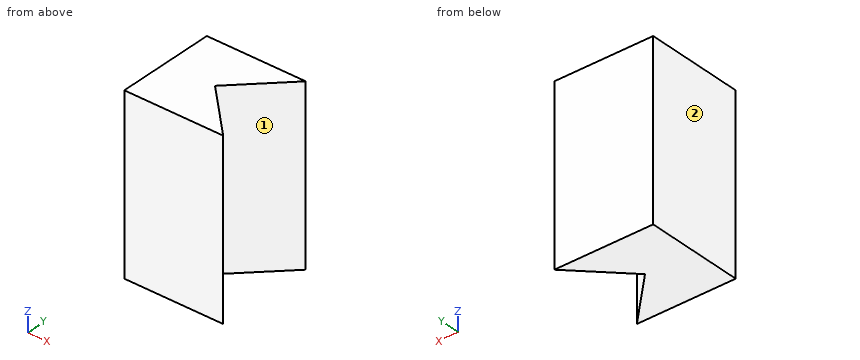
from build123d import *

# Parameters (mm, degrees)
F0_W     = 101.6
F0_H     = 101.6
F1_DEPTH = 177.8
F3_DEPTH = 177.8


with BuildPart() as f1:
    # F0 (on Top) → F1 (new body)
    with BuildSketch(Plane.XY):
        Rectangle(F0_W, F0_H)
    extrude(amount=F1_DEPTH)

    # F2 (on face) → F3 (cut, through all)
    with BuildSketch(Plane.XY.offset(177.8)):
        Polygon((50.8, 50.8), (0, 0), (50.8, -50.8), align=None)
    extrude(amount=-F3_DEPTH, mode=Mode.SUBTRACT)


solid = f1.part
Could you check a few things on this model? Use its own coordinates, in mm. Face numbers are marked on the shaded views. A direction names the side the tool comes from. Give positions to 0.01 mm unless a question says otherwise; leave off trailing zeros. Loops run counter-clockwise (first coordinate to the right, second up) from the corner with the lowest first, then second, coordinate; pieces in that order, holes last. Notation, with made-up numbers: (29, -9.75) -> (72, -9.75) arc R9 ccw to (72, -5.75) -> close; hole circle Ø7 at (-11.75, 66.25). An arc over 180 degrees is marked (long way). Return JSON: item names as keys, results as strings.
Item 1: I need wall thicknesses on L1, parallel to Y at x = 34, z = 125; L2, parallel to Y at x = 26, z = 78; L3, parallel to X at y = 40, z = 54.5. Which ranges of each line are inside material? Lowest first, please. Write a range as from..to.
Geometry results:
{"L1": "y = -50.8..-34, 34..50.8", "L2": "y = -50.8..-26, 26..50.8", "L3": "x = -50.8..40"}
Item 2: Which directions (+Z, -Z, +X, -X, +Y, -Y) give clear straight access to the entire face, cutting with the end or side of a thin tool? Please do the marked faces 1 and 2.
Geometry results:
{"face 1": "+Z, -Z, +X", "face 2": "+Z, -Z, -X, +Y, -Y"}
Item 3: If we section it at A-A on x = 43: List the corners of the cut face in (y, z) for me.
Geometry results:
{"outline": "(-50.8, 0) -> (-43, 0) -> (-43, 177.8) -> (-50.8, 177.8) -> close; (43, 0) -> (50.8, 0) -> (50.8, 177.8) -> (43, 177.8) -> close"}
Item 4: I'm going to push flat-ended pins straight in: pin 1 (3 mm diameter, centred on y = 27, z = 149.5, fed in from +X); pin 2 (10 mm diameter, centred on y = 12.5, z = 134, fed in from +X); pin 3 (6 mm diameter, centred on x = 30, y = 24, fed in from -Z). Where does each tip first touch, or does it pass through?
Geometry results:
{"pin 1": "stops at x = 28.5", "pin 2": "stops at x = 17.5", "pin 3": "passes through"}
Item 5: If we section it at C-C on y = 13: List the corners of the cut face in (x, z) for me.
Geometry results:
{"outline": "(-50.8, 0) -> (13, 0) -> (13, 177.8) -> (-50.8, 177.8) -> close"}
Item 6: If we section it at B-B on z = 75.5: List the corners of the cut face in (x, y) for me, plus the area to 3 significant figures.
Geometry results:
{"outline": "(-50.8, -50.8) -> (50.8, -50.8) -> (0, 0) -> (50.8, 50.8) -> (-50.8, 50.8) -> close", "area": "7,740 mm²"}
Item 7: If we section it at D-D on y = -15: List the corners of the cut face in (x, z) for me, plus the area to 3 significant figures.
Geometry results:
{"outline": "(-50.8, 0) -> (15, 0) -> (15, 177.8) -> (-50.8, 177.8) -> close", "area": "11,700 mm²"}
